from build123d import *

# Parameters (mm, degrees)
SKETCH1_W                        = 425.45
SKETCH1_H                        = 44.45
BASE_FLANGE1_DEPTH               = 4.2672
EDGE_FLANGE1_STRIP_CUT_DEPTH     = 425.45
EDGE_FLANGE1_DEPTH               = 425.45
EDGE_FLANGE1_START               = 4.2672
EDGE_FLANGE1_PROFILE_W           = 504.825
EDGE_FLANGE1_PROFILE_H           = 49.905487105
EDGE_FLANGE1_FLAT_DEPTH          = 4.2672
EDGE_FLANGE2_STRIP_CUT_DEPTH     = 425.45
EDGE_FLANGE2_DEPTH               = 425.45
CHAMFER1_SIZE                    = 6.35
F_17_64_0_26563_DIAMETER_HOLE1_D = 6.747002


# Sheet-metal steps are written as plain solids
with BuildPart() as part:
    # Sketch1 → Base-Flange1 (new body)
    with BuildSketch(Plane(origin=(0, 0, 0), x_dir=(1, 0, 0), z_dir=(0, 1, 0))):
        Rectangle(SKETCH1_W, SKETCH1_H)
    extrude(amount=-BASE_FLANGE1_DEPTH)

    # Edge-Flange1 strip (across the edge) → Edge-Flange1 strip cut (cut)
    with BuildSketch(Plane(origin=(212.725, -4.2672, 22.225), x_dir=(0, -0.96592582628907, -0.2588190451025146), z_dir=(-1, 0, 0))):
        Polygon((-9.522131081, 19.049882248), (-4.052559965, -1.362835054), (0.069238721, -0.258402425), (-5.400332395, 20.154314877), align=None)
    extrude(amount=EDGE_FLANGE1_STRIP_CUT_DEPTH, mode=Mode.SUBTRACT)

    # Edge-Flange1 bend section (across the edge) → Edge-Flange1 (add)
    with BuildSketch(Plane(origin=(212.725, -4.2672, 22.225), x_dir=(0, -0.96592582628907, -0.2588190451025146), z_dir=(-1, 0, 0))):
        with BuildLine():
            Line((-4.2672, 0.267517875), (0, 0.267517875))
            ThreePointArc((0, 0.267517875), (0.017384042, 0.002288653), (0.069238721, -0.258402425))
            Line((0.069238721, -0.258402425), (-4.052559965, -1.362835054))
            ThreePointArc((-4.052559965, -1.362835054), (-4.213309471, -0.554692715), (-4.2672, 0.267517875))
        make_face()
    extrude(amount=EDGE_FLANGE1_DEPTH)

    # Edge-Flange1 profile (on flange) → Edge-Flange1 flat (add)
    with BuildSketch(Plane(origin=(0, -4.2672, 22.225), x_dir=(-1, 0, 0), z_dir=(0, 0.96592582628907, 0.2588190451025146)).offset(EDGE_FLANGE1_START)):
        with Locations((0, 25.220261428)):
            Rectangle(EDGE_FLANGE1_PROFILE_W, EDGE_FLANGE1_PROFILE_H)
    extrude(amount=-EDGE_FLANGE1_FLAT_DEPTH)

    # Edge-Flange2 strip (across the edge) → Edge-Flange2 strip cut (cut)
    with BuildSketch(Plane(origin=(-212.725, -4.2672, -22.225), x_dir=(0, -0.9961946980917461, 0.08715574274765156), z_dir=(1, 0, 0))):
        Polygon((-6.085074523, 20.592090897), (-4.243229642, -0.460292419), (0.007732373, -0.088381433), (-1.834112507, 20.964001883), align=None)
    extrude(amount=EDGE_FLANGE2_STRIP_CUT_DEPTH, mode=Mode.SUBTRACT)

    # Edge-Flange2 section (across the edge) → Edge-Flange2 (add)
    with BuildSketch(Plane(origin=(-212.725, -4.2672, -22.225), x_dir=(0, -0.9961946980917461, 0.08715574274765156), z_dir=(1, 0, 0))):
        with BuildLine():
            Line((-4.2672, 0.088719036), (-4.2672, 50.38333524))
            Line((-4.2672, 50.38333524), (0, 50.38333524))
            Line((0, 50.38333524), (0, 0.088719036))
            ThreePointArc((0, 0.088719036), (0.001934014, 8.4441e-05), (0.007732373, -0.088381433))
            Line((0.007732373, -0.088381433), (-4.243229642, -0.460292419))
            ThreePointArc((-4.243229642, -0.460292419), (-4.261204557, -0.186048209), (-4.2672, 0.088719036))
        make_face()
    extrude(amount=EDGE_FLANGE2_DEPTH)

    # Chamfer1
    chamfer1_edges = [part.edges().sort_by_distance(p)[0] for p in [
        (-252.4125, -2.275539378, 23.035618739),
        (252.4125, -2.275539378, 23.035618739),
        (252.4125, -15.192029896, 71.240617608),
        (-252.4125, -15.192029896, 71.240617608),
        (-212.725, -6.532915997, -72.602566931),
        (212.725, -6.532915997, -72.602566931),
    ]]
    chamfer(chamfer1_edges, length=CHAMFER1_SIZE)

    # 17/64 (0.26563) Diameter Hole1 (through all)
    with Locations(Plane(origin=(0, 5.696696884, 1.52642533), x_dir=(1, 0, 0), z_dir=(0, 0.96592582628907, 0.2588190451025147))):
        with Locations((-240.50625, -35.539651994), (-240.50625, -60.939651994), (240.50625, -60.939651994), (240.50625, -35.539651994)):
            Hole(F_17_64_0_26563_DIAMETER_HOLE1_D / 2)


solid = part.part
Work out the finished part from the listing and answer in its coordinate system (mm). A direction names the side the tool comes from. Round coordinates to 2 decimals unless told otherwise and drop trailing zeros. Write each loop counter-clockwise with the first axis right and the second up, starting at its lowest first coordinate (ties: lowest second). Pieces come first, ordered by that corner, then holes. Notation, with made-up numbers: (48.25, -21) -> (54.25, -21) arc R19 cw to (54.25, 11) -> close; hole circle Ø8 at (15, -6.75). An arc over 180 degrees is marked (long way). Write each question's results on one line, items separated by ' | '.
Item 1: The mould has two halves that part along Z. Classify faces 3 (the face through (3.534, -10.885, 46.923)), 4 (the face through (-3, 0, 0)), 5 (the face through (-2.978, -2.185, -47.386)): +Z half, -Z half, draft (parallel to the pull), parting line (faces both ways), or undercut.
Result set:
face 3: undercut | face 4: draft | face 5: -Z half
Item 2: A cutting plane is placed at B-B, the plane z = 49.5. Determine the outline of the cut face in (x, y).
Result set:
outline: (-252.41, -11.58) -> (252.41, -11.58) -> (252.41, -7.16) -> (-252.41, -7.16) -> close
Item 3: Find the intervals of material crossed by line 1 along X through (y, z) = (-5.5, -42.5) (3 decimals); line 2 along Y through (x, z) = (-36, -23.5); line 3 along Y through (x, z) = (-76.5, -43), in increasing order. Write a range as [from, to].
Result set:
line 1: [-212.725, 212.725] | line 2: [-4.38, -0.1] | line 3: [-6.08, -1.8]
Item 4: Flat-ended cylindrical pins translate along their axes: P1, Ø4, axis at y = -4.5, z = -2, coming from the +X side (3 decimals); P2, Ø9, axis at y = -6, z = -38, coming from the -X side (3 decimals); P3, Ø3, axis at x = 85, z = 51.5, coming from the +Y side. Find the tip coordinate at first contact, or state that the pin passes through.
Result set:
P1: x = 212.725 | P2: x = -212.725 | P3: y = -7.29
Item 5: Which of the six approach directions +Z, -Z, +X, -X, +Y, -Y give full straight-line access (tool end or side, diameter ignored) to faces 1 (the face through (-3, -4.267, 0)), 2 (the face through (3.534, -6.763, 48.028))?
Result set:
face 1: +X, -X, -Y | face 2: +Z, +X, -X, +Y
Item 6: A cutting plane is placed at A-A, the plane x = 78. Determine the outline of the cut face in (y, z).
Result set:
outline: (-17.25, 70.69) -> (-4.34, 22.48) arc R2.03 cw to (-4.27, 21.96) -> (-4.27, -22.14) arc R2.03 cw to (-4.27, -22.31) -> (-8.66, -72.42) -> (-4.41, -72.79) -> (-0.02, -22.69) arc R6.3 ccw to (0, -22.14) -> (0, 21.96) arc R6.3 ccw to (-0.21, 23.59) -> (-13.13, 71.79) -> close
